The drawing under review shows one solid part. Ordinate dimensions are in mm from its lowest x, y, z. Give positions to 0.01 mm unless a question says otherwise; leave off trailing zeros. Order: outer loops, then holes, each group sorted by start corner. A loop starts at its lowest first (then second) coordinate and runs counter-clockwise, first axis right, second up. Notation, with made-up numbers: (32.5, 63.25) -> (75.5, 63.25) arc R20 cw to (75.5, 87.25) -> close; hole circle Ø2 at (40, 31.25). An arc over 180 degrees is marked (long way). Return JSON: item names as keys, results as strings. Group by question number.
1) To check wall thickness, follow line 1 along X through (y, z) = (8.75, 0.1) (3 decimals); line 2 along X through (y, z) = (5.25, 1.4); line 3 along Y through (x, z) = (11.75, 0.75). State the ranges of each line that lie inside material, in increasing order.
2) Add section B-B (z = 0.6). Give the boundary of the cut face in (x, y) (3 decimals).
3) Add section A-A (y = 4.75). Give the boundary of the cut face in (x, z) (1 decimal), then the cut area to 3 significant figures.
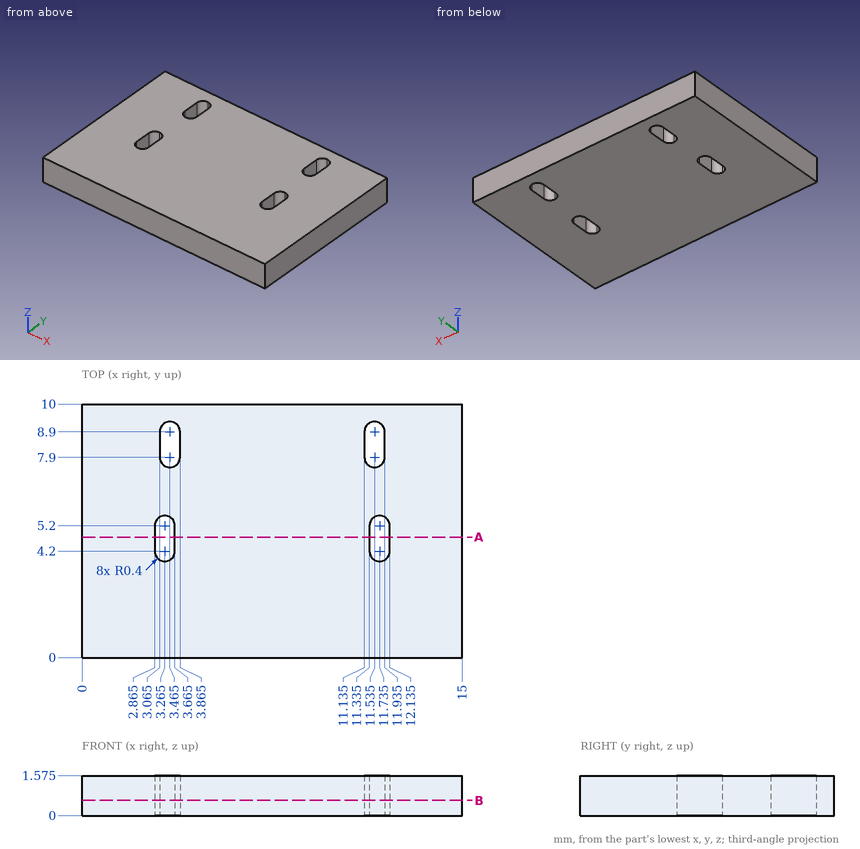
Evaluation:
{
 "1": {"line 1": "0 to 3.065, 3.865 to 11.135, 11.935 to 15", "line 2": "0 to 2.87, 3.66 to 11.34, 12.13 to 15", "line 3": "0 to 3.8, 5.6 to 7.56, 9.24 to 10"},
 "2": {"outline": "(0, 0) -> (15, 0) -> (15, 10) -> (0, 10) -> close; hole (2.865, 4.2) arc R0.4 ccw to (3.665, 4.2) -> (3.665, 5.2) arc R0.4 ccw to (2.865, 5.2) -> close; hole (3.065, 7.9) arc R0.4 ccw to (3.865, 7.9) -> (3.865, 8.9) arc R0.4 ccw to (3.065, 8.9) -> close; hole (11.135, 7.9) arc R0.4 ccw to (11.935, 7.9) -> (11.935, 8.9) arc R0.4 ccw to (11.135, 8.9) -> close; hole (11.335, 4.2) arc R0.4 ccw to (12.135, 4.2) -> (12.135, 5.2) arc R0.4 ccw to (11.335, 5.2) -> close"},
 "3": {"outline": "(0, 0) -> (2.9, 0) -> (2.9, 1.6) -> (0, 1.6) -> close; (3.7, 0) -> (11.3, 0) -> (11.3, 1.6) -> (3.7, 1.6) -> close; (12.1, 0) -> (15, 0) -> (15, 1.6) -> (12.1, 1.6) -> close", "area": "21.1 mm^2"}
}
